Part print with two shaded views. Sizes in mm from the minimum x, y, z corner. A direction names the side the tool comes from. Coordinates: 2 decimals unless noted, no trailing zeros. Order: outer loops, then holes, each group sorted by start corner. A loop starts at its lowest first (then second) coordinate and runs counter-clockwise, first axis right, second up.
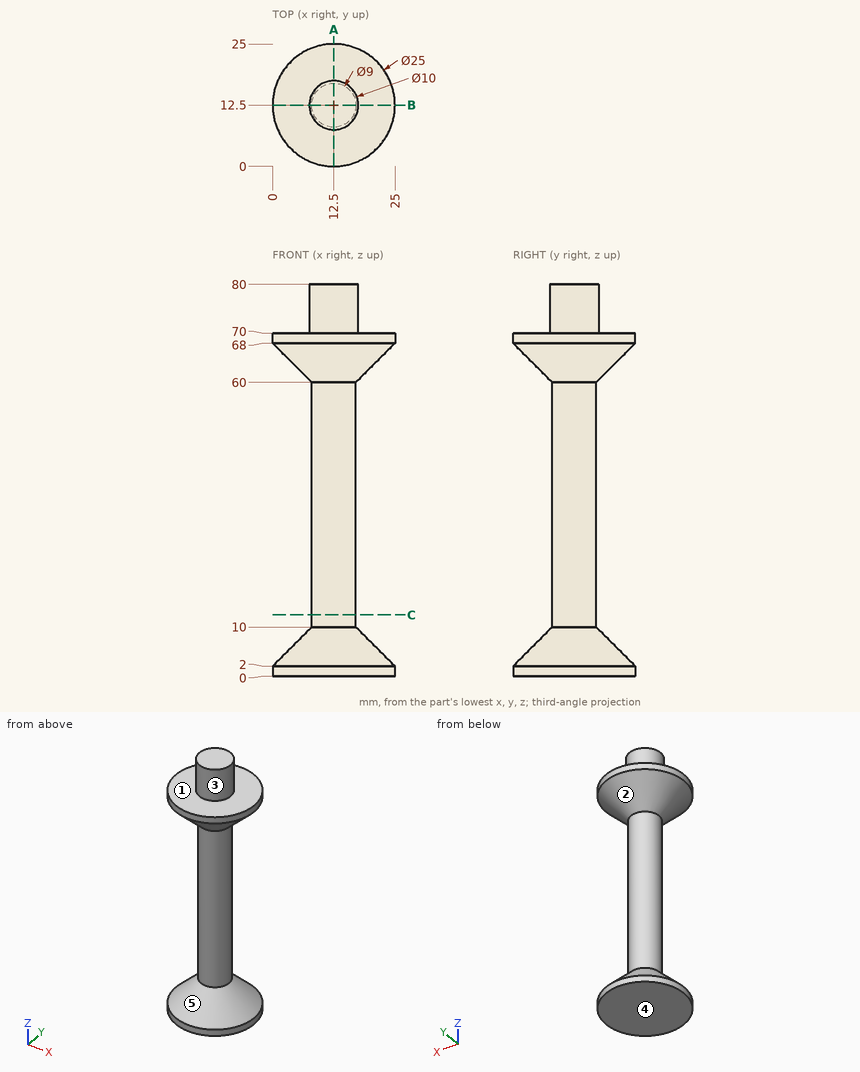
Q1. Cut at C-C on z = 12.5. Write the cut outline in (x, y).
Results list:
outline: circle Ø9 at (12.5, 12.5)
Q2. Which spindle directions (+Z, -Z, +X, -X, +Y, -Y) get a long thin tool onto all of the face, cutting with end or side? Do the marked faces 4 and 5. Say none if no direction does.
Results list:
face 4: -Z, +X, -X, +Y, -Y
face 5: none
Q3. Pin check, flat tips, straight feed: pin 1 Ø8 at (y, z) = (11, 46.5) entering from +X; pin 2 Ø1.5 at (y, z) = (17, 66.5) entering from -X; pin 3 Ø5 at (y, z) = (3.5, 52.5) entering from -X; pin 4 Ø5 at (y, z) = (14, 59.5) entering from +X. Stop position of each tip, or through.
Results list:
pin 1: stops at x = 17
pin 2: stops at x = 1.59
pin 3: passes through
pin 4: stops at x = 18.87
Q4. Mould opens along Z. For the marked faces 1, 2 and 3 say: pulls with the +Z half, pulls with the -Z half, needs draft (parallel to the pull), parting line crosses it, or undercut.
Results list:
face 1: pulls with the +Z half
face 2: undercut
face 3: needs draft
Q5. Wall check: line 1 along Z through (x, y) = (3.5, 11.25); line 2 along Z through (x, y) = (20.5, 13.5); line 3 along X through (y, z) = (15, 62.5). Give the ranges that are in metal, low to high.
Results list:
line 1: z = 0 to 5.41, 64.59 to 70
line 2: z = 0 to 6.44, 63.56 to 70
line 3: x = 5.96 to 19.04
Q6. Cut at A-A on x = 12.5. Write the cut outline in (y, z), and give its area (3 significant figures).
Results list:
outline: (0, 0) - (25, 0) - (25, 2) - (17, 10) - (17, 60) - (25, 68) - (25, 70) - (17.5, 70) - (17.5, 80) - (7.5, 80) - (7.5, 70) - (0, 70) - (0, 68) - (8, 60) - (8, 10) - (0, 2) - close
area: 922 mm2
